Build history of the part. All positions in model axes, mm. A direction names the side the tool comes from. Give positions to 0.01 mm unless a question says otherwise; leave off trailing zeros. Loops run counter-clockwise (first coordinate to the right, second up) from the corner with the lowest first, then second, coordinate; pieces in that order, holes last. Notation, with made-up numbers: (71, -2) -> (125, -2) arc R26 ccw to (125, 18) -> close; hole circle Ø3 at (-12, 11.5). An arc over 180 degrees is marked (long way). Answer in a Markdown table with one row per item. Add a question column.
from build123d import *

# Parameters (mm, degrees)
F0_W     = 53.975
F0_H     = 38.1
F1_DEPTH = 127


with BuildPart() as f1:
    # F0 (on Front) → F1 (new body)
    with BuildSketch(Plane.XZ):
        Polygon((0, -12.7), (0, 0), (-25.4, 0), (-25.4, -12.7), (-57.15, -12.7), (-57.15, 0), (-76.2, 0), (-107.95, -54.992613), (-75.735204, -109.985226), (-56.685204, -109.985226), (-56.685204, -97.285226), (-25.4, -97.285226), (-25.4, -109.985226), (0, -109.985226), (0, -97.285226), (31.75, -97.285226), (31.75, -109.985226), (50.8, -109.985226), (82.55, -54.992613), (50.8, 0), (31.75, 0), (31.75, -12.7), align=None)
        with Locations((-52.3875, -57.15)):
            Rectangle(F0_W, F0_H, mode=Mode.SUBTRACT)
        with Locations((26.9875, -57.15)):
            Rectangle(F0_W, F0_H, mode=Mode.SUBTRACT)
    extrude(amount=F1_DEPTH)


solid = f1.part
(1) Saw through at A-A, the plane y = -19. State how many separate pieces and enclosed holes the cut face has, then the cut area to 3 significant figures.
(2) Saw through at C-C, the plane z = -59. List the corners of the cut face in (x, y) (3 decimals).
(3) 3-axis set-ups, long thin cutter, end or side, ignore diameter. For faces 1 (the flat face through (-41, -63, -97.285)), 2 (the flat face through (16, -63, -12.7)), 3 (the flat face through (-25.4, -63, -57)): which of +Z, -Z, +X, -X, +Y, -Y reach the whole face in a straight line?
(4) Flat gauge pins, fed straight in: pin 1 Ø10 at (y, z) = (-62.5, -101) entering from +X; pin 2 Ø10 at (y, z) = (-36.5, -103.5) entering from -X; pin 3 Ø1.5 at (y, z) = (-38.5, -79.5) entering from -X. Where does each tip first touch, or does it go through?
(5) Saw through at D-D, the plane z = -47. List the corners of the cut face in (x, y) (3 decimals).
(6) Saw through at B-B, the plane x = 28. List the corners of the cut face in (y, z).
(7) Two-plate mould, pull along X, no slides. Class faces 4 (the flat face through (-57.15, -63, -6)), 5 (the flat face through (41, -63, 0)), 6 (the flat face through (-91.85, -62.61, -27.11)): released by +X, released by -X, zero draft, split by the parting line, or undercut.
(8) Wall check: line 1 along X through (y, z) = (-119, -55) (3 decimals); line 2 along Z through (x, y) = (-60.5, -85.5); line 3 along X through (y, z) = (-66, -11.5). Give the ranges that are in metal, low to high. Write a range as from..to.
Worked answers:
| question | item | result |
|---|---|---|
| 1 | separate pieces | 1 |
| 1 | enclosed holes | 2 |
| 1 | area | 11,700 mm^2 |
| 2 | outline | (-105.602, -127) -> (-79.375, -127) -> (-79.375, 0) -> (-105.602, 0) -> close; (-25.4, -127) -> (0, -127) -> (0, 0) -> (-25.4, 0) -> close; (53.975, -127) -> (80.236, -127) -> (80.236, 0) -> (53.975, 0) -> close |
| 3 | face 1 | -Z, +Y, -Y |
| 3 | face 2 | +Z, +Y, -Y |
| 3 | face 3 | +Y, -Y |
| 4 | pin 1 | x = 58.87 |
| 4 | pin 2 | x = -82.46 |
| 4 | pin 3 | x = -94.03 |
| 5 | outline | (-103.335, -127) -> (-79.375, -127) -> (-79.375, 0) -> (-103.335, 0) -> close; (-25.4, -127) -> (0, -127) -> (0, 0) -> (-25.4, 0) -> close; (53.975, -127) -> (77.935, -127) -> (77.935, 0) -> (53.975, 0) -> close |
| 6 | outline | (-127, -97.29) -> (0, -97.29) -> (0, -76.2) -> (-127, -76.2) -> close; (-127, -38.1) -> (0, -38.1) -> (0, -12.7) -> (-127, -12.7) -> close |
| 7 | face 4 | undercut |
| 7 | face 5 | zero draft |
| 7 | face 6 | released by -X |
| 8 | line 1 | -107.946..-79.375, -25.4..0, 53.975..82.546 |
| 8 | line 2 | -109.99..-76.2, -38.1..0 |
| 8 | line 3 | -82.84..-57.15, -25.4..0, 31.75..57.44 |
